Design review of the part built by this model. Coordinates are the model's own, in mm. Coordinates: 2 decimals unless noted, no trailing zeros. Loops run counter-clockwise (first coordinate to the right, second up) from the corner with the lowest first, then second, coordinate; pieces in that order, holes last. Notation, with made-up numbers: M 58.25,74 L 82.25,74 A28 cw 82.25,113 Z; hole C 15.5,-13.75 d2. An arc over 180 degrees is marked long. One line per item, written item: value.
```python
from build123d import *

# Parameters (mm, degrees)
SKETCH1_W            = 25
SKETCH1_H            = 97
BOSS_EXTRUDE1_DEPTH  = 3
SKETCH4_W            = 10
SKETCH4_H            = 15
CUT_EXTRUDE1_DEPTH   = 170.215838502
FILLET2_R            = 1
M4_CLEARANCE_HOLE1_D = 4.5


with BuildPart() as part:
    # Sketch1 → Boss-Extrude1 (new body)
    with BuildSketch(Plane(origin=(0, 0, 0), x_dir=(1, 0, 0), z_dir=(0, 1, 0))):
        with BuildLine():
            Line((-45, -10), (-10, -10))
            Line((-10, -10), (-10, -33))
            ThreePointArc((-10, -33), (0, -43), (10, -33))
            Line((10, -33), (10, 117))
            ThreePointArc((10, 117), (7.071067812, 124.071067812), (0, 127))
            Line((0, 127), (-35, 127))
            Line((-35, 127), (-35, 150))
            ThreePointArc((-35, 150), (-45, 160), (-55, 150))
            Line((-55, 150), (-55, 0))
            ThreePointArc((-55, 0), (-52.071067812, -7.071067812), (-45, -10))
        make_face()
        with Locations((-22.5, 58.5)):
            Rectangle(SKETCH1_W, SKETCH1_H, mode=Mode.SUBTRACT)
    extrude(amount=BOSS_EXTRUDE1_DEPTH)

    # Sketch4 → Cut-Extrude1 (cut, through all)
    with BuildSketch(Plane(origin=(0, 3, 0), x_dir=(1, 0, 0), z_dir=(0, 1, 0))):
        with Locations((-45, 99.5)):
            Rectangle(SKETCH4_W, SKETCH4_H)
        with Locations((0, 66.5)):
            Rectangle(SKETCH4_W, SKETCH4_H)
    extrude(amount=-CUT_EXTRUDE1_DEPTH, mode=Mode.SUBTRACT)

    # Fillet2
    fillet2_edges = [part.edges().sort_by_distance(p)[0] for p in [
        (-35, 1.5, -127),
        (-10, 1.5, 10),
        (-35, 1.5, -107),
        (-35, 1.5, -10),
        (-10, 1.5, -10),
        (-10, 1.5, -107),
        (-50, 1.5, -92),
        (-50, 1.5, -107),
        (-40, 1.5, -107),
        (-40, 1.5, -92),
        (-5, 1.5, -59),
        (-5, 1.5, -74),
        (5, 1.5, -74),
        (5, 1.5, -59),
    ]]
    fillet(fillet2_edges, radius=FILLET2_R)

    # M4 Clearance Hole1 (through all)
    with Locations(Plane(origin=(0, 3, 0), x_dir=(1, 0, 0), z_dir=(0, 1, 0))):
        with Locations((-43.5, 150), (1.5, 117), (-43.5, 0), (1.5, -33)):
            Hole(M4_CLEARANCE_HOLE1_D / 2)


solid = part.part
```
(1) Insertion check: pin 1 (0.9 mm diameter, centred on x = -21, y = 2, fed in from -Z); pin 2 (1.5 mm diameter, centred on x = -25.5, y = 1.5, fed in from +Z). Each pin has a flat end and moves straight along its axis. Give the tip position at first contact, or say it passes through.
Reply:
pin 1: stops at z = -127
pin 2: stops at z = 10
(2) We need section A-A on x = -17. State the section outline as (y, z) points, then the cut area to 3 significant figures.
Reply:
outline: M 0,-127 L 3,-127 L 3,-107 L 0,-107 Z; M 0,-10 L 3,-10 L 3,10 L 0,10 Z
area: 120 mm2
(3) To check wall thickness, follow line 1 along X through (y, z) = (2.1, -71.5); line 2 along X through (y, z) = (2.3, -25); line 3 along Z through (x, y) = (1.5, 0.8). State the ranges of each line that lie inside material, in increasing order. Write a range as [from, to].
Reply:
line 1: x = [-55, -35], [-10, -5], [5, 10]
line 2: x = [-55, -35], [-10, 10]
line 3: z = [-126.89, -119.25], [-114.75, -74], [-59, 30.75], [35.25, 42.89]
(4) We need section B-B on y = 2.3. State how many separate pieces and enclosed holes the cut face has, then the cut area to 3 significant figures.
Reply:
separate pieces: 1
enclosed holes: 7
area: 7,310 mm2
(5) Mouldability with a two-part tool opening along Z and no side actions: class faces 1 (the cylindrical face through (0, 1, 43)), 2 (the cylindrical face through (-45, 1, -160)), 3 (the cylindrical face through (-41.252, 1.479, -0.099)), 4 (the cylindrical face through (1.988, 1.479, -114.804)) as released by +Z, released by -Z, zero draft, split by the parting line, or undercut.
Reply:
face 1: released by +Z
face 2: released by -Z
face 3: undercut
face 4: undercut
